Autodesk Inventor part; units mm, degrees
ref_plane "YZ Plane" through (0, 0, 0) normal (1, 0, 0) x (0, 1, 0)
ref_plane "XZ Plane" through (0, 0, 0) normal (0, 1, 0) x (-1, 0, 0)
ref_plane "XY Plane" through (0, 0, 0) normal (0, 0, 1) x (1, 0, 0)
sketch "Sketch1" plane through (0, 0, 0) normal (0, 0, 1) x (1, 0, 0)
  line L0 (17, -10) -> (-17, -10)
  line L1 (-17, -10) -> (-17, 10)
  line L2 (-17, 10) -> (17, 10)
  line L3 (17, 10) -> (17, -10)
  line L4 (17, -10) -> (-17, 10) construction
  line L5 (-17, -10) -> (17, 10) construction
  point P0 (0, 0)
extrude "Extrusion1" add sketch "Sketch1" along normal blind 1
sketch "Sketch2" plane through (0, 0, 1) normal (0, 0, 1) x (1, 0, 0)
  line L0 (10, -7) -> (-10, -7)
  line L1 (-10, -7) -> (-10, 7)
  line L2 (-10, 7) -> (10, 7)
  line L3 (10, 7) -> (10, -7)
  line L4 (10, -7) -> (-10, 7) construction
  line L5 (-10, -7) -> (10, 7) construction
  point P0 (0, 0)
extrude "Extrusion2" add sketch "Sketch2" along normal blind 2
sketch "Sketch3" plane through (0, 0, 3) normal (0, 0, 1) x (1, 0, 0)
  circle A0 centre (0, 0) radius 7.0711
extrude "Extrusion3" add sketch "Sketch3" along normal blind 5
fillet "Fillet1" radius 5 1 edges at (-7.0711, 0, 8)
sketch "Sketch4" plane through (0, 0, 0) normal (0, 0, -1) x (-1, 0, 0)
  line L0 (16, -9) -> (15.5, -9)
  line L1 (15.5, -9) -> (15.5, -8.44)
  line L2 (15.5, -8.44) -> (16, -8.44)
  line L3 (16, -8.44) -> (16, -9)
  point P0 (0, 0)
  dimension "d7" = 0.5
  dimension "d8" = 0.56
extrude "Extrusion4" add sketch "Sketch4" along normal blind 2
mirror "Mirror1" about plane through (0, 0, 0) normal (1, 0, 0) of "Extrusion4"
mirror "Mirror2" about plane through (0, 0, 0) normal (0, 1, 0) of "Extrusion4", "Mirror1"
sketch "Sketch5" plane through (0, 0, -2) normal (0, 0, -1) x (-1, 0, 0)
  circle A0 centre (15.75, -8.7479) radius 1
  point P0 (0, 0)
  dimension "d11" = 2
extrude "Extrusion5" add sketch "Sketch5" along normal blind 2
sketch "Sketch6" plane through (-15.75, -8.7479, -4) normal (0, 0, -1) x (-1, 0, 0)
  line L0 (-0.25, 0.25) -> (0.25, 0.25)
  line L1 (0.25, 0.25) -> (0.25, -0.25)
  line L2 (0.25, -0.25) -> (-0.25, -0.25)
  line L3 (-0.25, -0.25) -> (-0.25, 0.25)
  line L4 (-0.25, 0.25) -> (0.25, -0.25) construction
  line L5 (0.25, 0.25) -> (-0.25, -0.25) construction
  point P0 (-15.75, 8.7479)
  point P1 (0, 0)
  dimension "d14" = 0.5
  dimension "d15" = 0.5
extrude "Extrusion6" add sketch "Sketch6" along normal blind 1
mirror "Mirror3" about plane through (0, 0, 0) normal (1, 0, 0) of "Extrusion6"
mirror "Mirror4" about plane through (0, 0, 0) normal (1, 0, 0) of "Extrusion6", "Extrusion5"
mirror "Mirror5" about plane through (0, 0, 0) normal (0, 1, 0) of "Extrusion5", "Extrusion6", "Mirror4"
sketch "Sketch7" plane through (0, 0, 1) normal (0, 0, 1) x (1, 0, 0)
  point P0 (0, 0)
ref_plane "Work Plane1" through (0, 0, 0) normal (0, 1, 0) x (-1, 0, 0)
properties part number "pir sensor"
For this review, take the finished solid that the model builds, in its own axes (mm). A direction names the side the tool comes from. Round coordinates to 2 decimals unless told otherwise and drop trailing zeros. Order: outer loops, then holes, each group sorted by start corner. A loop starts at its lowest first (then second) coordinate and runs counter-clockwise, first axis right, second up. Notation, with made-up numbers: M 39,15 L 45,15 A17 ccw 45,41 Z; hole C -8,-1 d3. An arc over 180 degrees is marked long. Use a Markdown table: item, result. Add a question column.
Item 1: Add section A-A, the plane x = -7.5. Give the boundary of the cut face in (y, z).
Item 2: Add section D-D, the plane x = 11.5. Give the boundary of the cut face in (y, z).
Item 3: To check wall thickness, follow line 1 along Z through (x, y) = (7, -3); line 2 along Z through (x, y) = (-12, -3.5); line 3 along Y through (x, z) = (-3, 1.5). State the ranges of each line that lie inside material, in increasing order.
Item 4: Add section C-C, the plane z = 2.5. Give the boundary of the cut face in (x, y).
Item 5: Add section B-B, the plane z = -2.75. Give the boundary of the cut face in (x, y).
Item 6: Mouldability with a two-part tool opening along Z and no side actions: class faces 6 (the flat face through (15.7, 9.2, -2)), 7 (the flat face through (7.4, 0.1, 3)), 8 (the cylindrical face through (16.704, -8.448, -2.986)) as released by +Z, released by -Z, zero draft, split by the parting line, or undercut.
Item 7: Tool access review of faces 1 (the flat face through (-10, 0, 2)), 2 (the cylindrical face through (-16.704, 8.448, -2.986)), 3 (the flat face through (0.2, -10, 0.5)), 4 (the flat face through (-15.8, 9.2, -2)), 5 (the flat face through (10, 0, 2)): name each direction out of +Z, -Z, +X, -X, +Y, -Y from which nothing blocks a thin tool from reaching the whole face with its end or side.
Item 8: Insertion check: pin 1 (4 mm diameter, centred on y = -4.5, z = 6.5, fed in from +X); pin 2 (3 mm diameter, centred on x = 9.5, y = 1, fed in from -Z); pin 3 (0.6 mm diameter, centred on x = 15.5, z = -1, fed in from +Y); pin 4 (1.5 mm diameter, centred on y = -6.5, z = -3, fed in from +X). Each pin has a flat end and moves straight along its axis. Give the tip position at first contact, or say it passes through.
Geometry results:
| question | item | result |
|---|---|---|
| 1 | outline | M -10,0 L 10,0 L 10,1 L 7,1 L 7,3 L -7,3 L -7,1 L -10,1 Z |
| 2 | outline | M -10,0 L 10,0 L 10,1 L -10,1 Z |
| 3 | line 1 | z = 0 to 3 |
| 3 | line 2 | z = 0 to 1 |
| 3 | line 3 | y = -7 to 7 |
| 4 | outline | M -10,-7 L 10,-7 L 10,7 L -10,7 Z |
| 5 | outline | C -15.75,-8.75 d2; C -15.75,8.75 d2; C 15.75,-8.75 d2; C 15.75,8.75 d2 |
| 6 | face 6 | undercut |
| 6 | face 7 | released by +Z |
| 6 | face 8 | zero draft |
| 7 | face 1 | +Z, -X, +Y, -Y |
| 7 | face 2 | -Z |
| 7 | face 3 | +Z, -Z, +X, -X, -Y |
| 7 | face 4 | none |
| 7 | face 5 | +Z, +X, +Y, -Y |
| 8 | pin 1 | stops at x = 5.85 |
| 8 | pin 2 | stops at z = 0 |
| 8 | pin 3 | stops at y = 9 |
| 8 | pin 4 | passes through |
